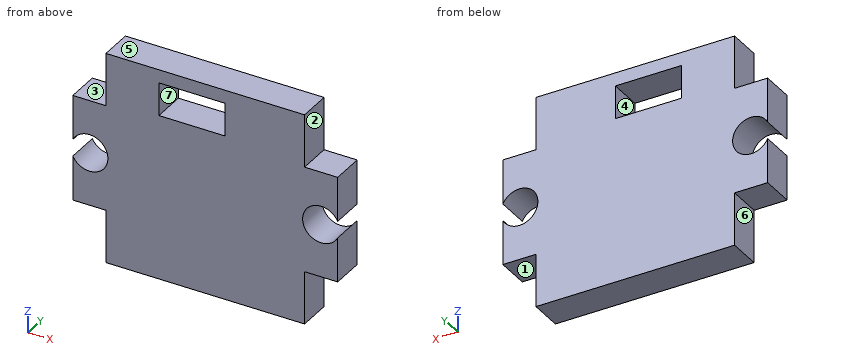
```python
from build123d import *

# Parameters (mm, degrees)
SKETCH1_W           = 25.4
SKETCH1_H           = 20.32
BOSS_EXTRUDE1_DEPTH = 3.175
SKETCH2_W           = 3.175
SKETCH2_H           = 5.08
CUT_EXTRUDE1_DEPTH  = 3.175
SKETCH3_R           = 1.778
CUT_EXTRUDE2_DEPTH  = 3.175
SKETCH4_W           = 6.35
SKETCH4_H           = 3.175
CUT_EXTRUDE3_DEPTH  = 3.175


with BuildPart() as part:
    # Sketch1 → Boss-Extrude1 (new body)
    with BuildSketch(Plane(origin=(0, 0, 0), x_dir=(1, 0, 0), z_dir=(0, 1, 0))):
        with Locations((12.7, -10.16)):
            Rectangle(SKETCH1_W, SKETCH1_H)
    extrude(amount=BOSS_EXTRUDE1_DEPTH)

    # Sketch2 → Cut-Extrude1 (cut)
    with BuildSketch(Plane(origin=(0, 3.175, 0), x_dir=(1, 0, 0), z_dir=(0, 1, 0))):
        with Locations((1.5875, -2.54)):
            Rectangle(SKETCH2_W, SKETCH2_H)
        with Locations((1.5875, -17.78)):
            Rectangle(SKETCH2_W, SKETCH2_H)
        with Locations((23.8125, -2.54)):
            Rectangle(SKETCH2_W, SKETCH2_H)
        with Locations((23.8125, -17.78)):
            Rectangle(SKETCH2_W, SKETCH2_H)
    extrude(amount=-CUT_EXTRUDE1_DEPTH, mode=Mode.SUBTRACT)

    # Sketch3 → Cut-Extrude2 (cut)
    with BuildSketch(Plane(origin=(0, 3.175, 0), x_dir=(1, 0, 0), z_dir=(0, 1, 0))):
        with Locations((1.5875, -10.16)):
            Circle(SKETCH3_R)
        with Locations((23.8125, -10.16)):
            Circle(SKETCH3_R)
    extrude(amount=-CUT_EXTRUDE2_DEPTH, mode=Mode.SUBTRACT)

    # Sketch4 → Cut-Extrude3 (cut)
    with BuildSketch(Plane(origin=(0, 3.175, 0), x_dir=(1, 0, 0), z_dir=(0, 1, 0))):
        with Locations((11.43, -17.4625)):
            Rectangle(SKETCH4_W, SKETCH4_H)
    extrude(amount=-CUT_EXTRUDE3_DEPTH, mode=Mode.SUBTRACT)


solid = part.part
```
Here's how the part is built. I have some questions about the finished solid (model axes, mm). Face numbers are marked on the shaded views. A direction names the side the tool comes from. Coordinates: 2 decimals unless noted, no trailing zeros. Order: outer loops, then holes, each group sorted by start corner. A loop starts at its lowest first (then second) coordinate and runs counter-clockwise, first axis right, second up.
1) Which directions (+Z, -Z, +X, -X, +Y, -Y) give clear straight access to the entire face, cutting with the end or side of a thin tool? Please do the marked faces 1, 2, 3 and 4.
2) Imagine slicing it at D-D on z = 3.25. List the corners of the cut face in (x, y) for me (3 decimals).
3) I need wall thicknesses on line 1 (X direction, y = 2.7, z = 17.25) (3 decimals); line 2 (Z direction, x = 12.5, y = 2.65) (3 decimals); line 3 (X direction, y = 2.05, z = 10.16). Which ranges of each line are inside material? Lowest first, please.
4) Will these pins go through, and if not, where does the flat tip stop? pin 1 (10 mm diameter, centred on x = 4, z = 10, fed in from -Y); pin 2 (1 mm diameter, centred on x = 2, y = 1.5, fed in from -Z); pin 3 (1.6 mm diameter, centred on y = 1, z = 18, fed in from +X) (3 decimals); pin 4 (1.6 mm diameter, centred on x = 24, y = 1, fed in from +Z).
5) We'd pull the mould along X, two halves only. Please class the marked faces 5, 6 and 7: +X half, -X half, draft (parallel to the pull), parting line (faces both ways), or undercut.
6) Imagine slicing it at A-A on x = 11.25. List the corners of the cut face in (y, z) for me (3 decimals).
7) Imagine slicing it at C-C on z = 10.16. List the corners of the cut face in (x, y) for me (1 decimal).
Response values:
1. face 1: -Z, +X, +Y, -Y
1. face 2: +Z, +X, +Y, -Y
1. face 3: +Z, -X, +Y, -Y
1. face 4: +Y, -Y
2. outline: (3.175, 0) - (22.225, 0) - (22.225, 3.175) - (3.175, 3.175) - close
3. line 1: x = 3.175 to 8.255, 14.605 to 22.225
3. line 2: z = 0 to 15.875, 19.05 to 20.32
3. line 3: x = 3.37 to 22.03
4. pin 1: stops at y = 0
4. pin 2: stops at z = 5.08
4. pin 3: stops at x = 22.225
4. pin 4: stops at z = 15.24
5. face 5: draft
5. face 6: -X half
5. face 7: undercut
6. outline: (0, 0) - (3.175, 0) - (3.175, 15.875) - (0, 15.875) - close; (0, 19.05) - (3.175, 19.05) - (3.175, 20.32) - (0, 20.32) - close
7. outline: (3.4, 0) - (22, 0) - (22, 3.2) - (3.4, 3.2) - close
